Design review of the part built by this model. Coordinates are the model's own, in mm. Round coordinates to 2 decimals unless told otherwise and drop trailing zeros. Loops run counter-clockwise (first coordinate to the right, second up) from the corner with the lowest first, then second, coordinate; pieces in that order, holes last. Notation, with made-up numbers: (-23.5, 38) - (8.5, 38) arc R31 ccw to (8.5, 67) - close; hole circle Ø2 at (77.5, -20.75). An arc over 180 degrees is marked (long way). Return JSON: item names as keys, results as strings. Group by question number.
(1) We need section B-B, the plane x = 0. Write out the cut boundary in (y, z) (3 decimals), and give its area (3 significant figures).
(2) Clearance check with a flat-ended pin moving along its axis: pin 1 (2 mm diameter, centred on x = 50, y = 1, fed in from +Z). State where the tip first meets the part, or that it passes through.
(3) We need section D-D, the plane z = 67.31. Write out the cut boundary in (x, y).
(4) Wall thickness on L1, parallel to Z at x = 35.5, y = 3.25; L2, parallel to Z at x = -11, y = 1; L3, parallel to Z at x = 32.5, y = 5: over which ranges is each line inside the solid? List them lowest first. Write a range as [from, to].
(5) We need section C-C, the plane y = 4.5. Give the number of separate pieces and of enclosed holes in the cut face, and give its area (3 significant figures).
(6) We need section A-A, the plane z = 0. Write out the cut boundary in (x, y) (3 decimals).
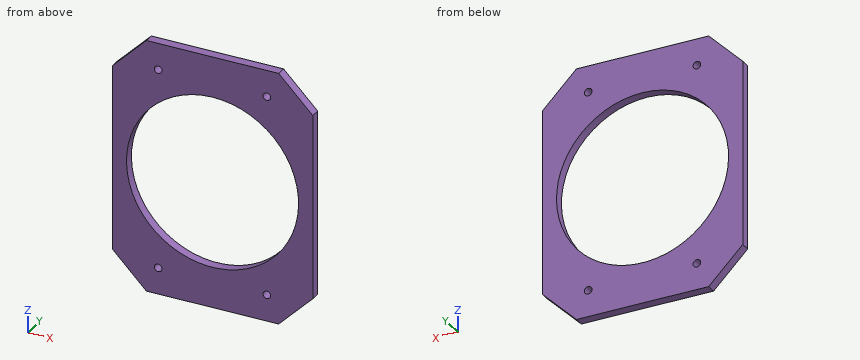
from build123d import *

# Parameters (mm, degrees)
BOSS_EXTRUDE1_DEPTH    = 6.35
F_10_CLEARANCE_HOLE1_D = 5.1054
CIRPATTERN1_COUNT      = 2
SKETCH4_R              = 57.785
CUT_EXTRUDE1_DEPTH     = 109.679651729


with BuildPart() as part:
    # Sketch1 → Boss-Extrude1 (new body)
    with BuildSketch(Plane(origin=(0, 0, 0), x_dir=(1, 0, 0), z_dir=(0, 1, 0))):
        Polygon((-67.31, 62.23), (-44.45, 85.09), (44.45, 85.09), (67.31, 62.23), (67.31, -62.23), (44.45, -85.09), (-44.45, -85.09), (-67.31, -62.23), align=None)
    extrude(amount=BOSS_EXTRUDE1_DEPTH)

    # 10 Clearance Hole1 (through all)
    with Locations(Plane(origin=(0, 6.35, 0), x_dir=(-1, 0, 0), z_dir=(0, 1, 0))):
        with Locations((36.5125, -67.31), (-36.5125, -67.31)):
            f_10_clearance_hole1 = Hole(F_10_CLEARANCE_HOLE1_D / 2)

    # CirPattern1: 10 Clearance Hole1 ×2 about axis
    cirpattern1_axis = Axis((0, 0, 0), (0, 1, 0))
    for i in range(1, CIRPATTERN1_COUNT):
        add(f_10_clearance_hole1.rotate(cirpattern1_axis, i * 360 / CIRPATTERN1_COUNT), mode=Mode.SUBTRACT)

    # Sketch4 → Cut-Extrude1 (cut, through all)
    with BuildSketch(Plane(origin=(0, 6.35, 0), x_dir=(1, 0, 0), z_dir=(0, 1, 0))):
        with Locations(Location((0, 0, 0), (0, 0, 270))):
            Circle(SKETCH4_R)
    extrude(amount=-CUT_EXTRUDE1_DEPTH, mode=Mode.SUBTRACT)


solid = part.part
Solutions:
{
 "1": {"outline": "(0, -85.09) - (6.35, -85.09) - (6.35, -57.785) - (0, -57.785) - close; (0, 57.785) - (6.35, 57.785) - (6.35, 85.09) - (0, 85.09) - close", "area": "347 mm^2"},
 "2": {"pin 1": "z = 80.54"},
 "3": {"outline": "(-62.23, 0) - (-39.07, 0) - (-39.07, 6.35) - (-62.23, 6.35) - close; (-33.96, 0) - (33.96, 0) - (33.96, 6.35) - (-33.96, 6.35) - close; (39.07, 0) - (62.23, 0) - (62.23, 6.35) - (39.07, 6.35) - close"},
 "4": {"L1": "[-85.09, -69.65], [-64.97, -45.59], [45.59, 64.97], [69.65, 85.09]", "L2": "[-85.09, -56.73], [56.73, 85.09]", "L3": "[-85.09, -47.78], [47.78, 85.09]"},
 "5": {"separate pieces": "1", "enclosed holes": "5", "area": "11,300 mm^2"},
 "6": {"outline": "(-67.31, 0) - (-57.785, 0) - (-57.785, 6.35) - (-67.31, 6.35) - close; (57.785, 0) - (67.31, 0) - (67.31, 6.35) - (57.785, 6.35) - close"}
}
